from build123d import *

# Parameters (mm, degrees)
F1_DEPTH = 5
F2_W     = 5
F2_H     = 40
F3_DEPTH = 12
F4_R     = 3
F5_R     = 1.5
F6_DEPTH = 10


with BuildPart() as f1:
    # F0 (on Top) → F1 (new body)
    with BuildSketch(Plane.XY):
        with BuildLine():
            ThreePointArc((-7.71248, 8.530396), (11.5, 0), (-7.71248, -8.530396))
            ThreePointArc((-7.71248, -8.530396), (-8.179899, -8.293039), (-8.703171, -8.324766))
            Line((-8.703171, -8.324766), (-13.541093, -9.959054))
            ThreePointArc((-13.541093, -9.959054), (-14.18276, -10.632379), (-13.992452, -11.54281))
            ThreePointArc((-13.992452, -11.54281), (2.75234, -17.929021), (16.810487, -6.814154))
            ThreePointArc((16.810487, -6.814154), (18.174589, -6.14164), (19.677769, -5.910335))
            Line((19.677769, -5.910335), (30.5, -5.910335))
            ThreePointArc((30.5, -5.910335), (34.035534, -7.374801), (35.5, -10.910335))
            Line((35.5, -10.910335), (35.5, -18))
            ThreePointArc((35.5, -18), (36.085786, -19.414214), (37.5, -20))
            Line((37.5, -20), (45.5, -20))
            Line((45.5, -20), (45.5, 0))
            Line((45.5, 0), (45.5, 20))
            Line((45.5, 20), (37.5, 20))
            ThreePointArc((37.5, 20), (36.085786, 19.414214), (35.5, 18))
            Line((35.5, 18), (35.5, 10.910335))
            ThreePointArc((35.5, 10.910335), (34.035534, 7.374801), (30.5, 5.910335))
            Line((30.5, 5.910335), (19.677769, 5.910335))
            ThreePointArc((19.677769, 5.910335), (18.174589, 6.14164), (16.810487, 6.814154))
            ThreePointArc((16.810487, 6.814154), (2.75234, 17.929021), (-13.992452, 11.54281))
            ThreePointArc((-13.992452, 11.54281), (-14.18276, 10.632379), (-13.541093, 9.959054))
            Line((-13.541093, 9.959054), (-8.703171, 8.324766))
            ThreePointArc((-8.703171, 8.324766), (-8.179899, 8.293039), (-7.71248, 8.530396))
        make_face()
    extrude(amount=F1_DEPTH)

    # F2 (on face) → F3 (join)
    with BuildSketch(Plane.XY.offset(5)):
        with Locations((43, 0)):
            Rectangle(F2_W, F2_H)
    extrude(amount=F3_DEPTH)

    # F4
    f4_edges = [f1.edges().sort_by_distance(p)[0] for p in [
        (40.5, 0, 5),
        (43, 20, 17),
        (43, -20, 17),
    ]]
    fillet(f4_edges, radius=F4_R)

    # F5 (on face) → F6 (cut)
    with BuildSketch(Plane(origin=(40.5, 0, 0), x_dir=(0, -1, 0), z_dir=(-1, 0, 0))):
        with Locations((-11.877556, 12)):
            Circle(F5_R)
        with Locations((11.877556, 12)):
            Circle(F5_R)
    extrude(amount=-F6_DEPTH, mode=Mode.SUBTRACT)


solid = f1.part
Geometry: final body of the model. Coordinates: model frame, mm. A direction names the side the tool comes from. Give positions to 0.01 mm unless a question says otherwise; leave off trailing zeros. Loops run counter-clockwise (first coordinate to the right, second up) from the corner with the lowest first, then second, coordinate; pieces in that order, holes last. Notation, with made-up numbers: (69, 3) -> (103, 3) arc R34 cw to (103, 33) -> close; hole circle Ø11 at (44, -17.75). An arc over 180 degrees is marked (long way). Put each result on its own line as item: value.
1. Pin query (flat end, axial travel): P1, Ø4, axis at x = 26, z = 2, coming from the -Y side; P2, Ø4, axis at y = 15.5, z = 3.5, coming from the -X side; P3, Ø10, axis at x = 26, y = 16, coming from the -Z side; P4, Ø4.5, axis at y = 9, z = 14, coming from the -X side. Return the tip coordinate at first contact, or that it passes through.
Taken from the geometry:
P1: stops at y = -5.91
P2: stops at x = -12.12
P3: passes through
P4: stops at x = 40.5
2. Cut plane C-C (y = 0). Return the cut outline in (x, z), plus the area to 3 significant figures.
Taken from the geometry:
outline: (11.5, 0) -> (45.5, 0) -> (45.5, 17) -> (40.5, 17) -> (40.5, 8) arc R3 cw to (37.5, 5) -> (11.5, 5) -> close
area: 232 mm2
3. Pull-direction query (X, two-part tool) for faces 5 (the cylindrical face through (34.07, 7.41, 2.46)), 6 (the cylindrical face through (39.64, 0.28, 5.9)), 7 (the cylindrical face through (42.965, 13.376, 12.066)); classes: released by +X, released by -X, zero draft, split by the parting line, or undercut.
Taken from the geometry:
face 5: undercut
face 6: released by -X
face 7: zero draft
4. Set-up query: faces 1 (the flat face through (42, -20, 7)), 2 (the flat face through (25, -5.91, 2)), 3 (the cylindrical face through (18.195, 6.135, 2.465)), 4 (the flat face through (-11.156, 9.153, 2.465)). Return all of +Z, -Z, +X, -X, +Y, -Y with unobstructed straight access to the full face (end or side cutting, diameter ignored); none if empty.
Taken from the geometry:
face 1: +Z, -Z, +X, -X, -Y
face 2: +Z, -Z, -Y
face 3: +Z, -Z, +Y
face 4: +Z, -Z, -X
5. Cut plane D-D (z = 2.25). Return the cut outline in (x, y).
Taken from the geometry:
outline: (-13.99, -11.54) arc R18.14 ccw to (16.81, -6.81) arc R5 cw to (19.68, -5.91) -> (30.5, -5.91) arc R5 cw to (35.5, -10.91) -> (35.5, -18) arc R2 ccw to (37.5, -20) -> (45.5, -20) -> (45.5, 20) -> (37.5, 20) arc R2 ccw to (35.5, 18) -> (35.5, 10.91) arc R5 cw to (30.5, 5.91) -> (19.68, 5.91) arc R5 cw to (16.81, 6.81) arc R18.14 ccw to (-13.99, 11.54) arc R1 ccw to (-13.54, 9.96) -> (-8.7, 8.32) arc R1 ccw to (-7.71, 8.53) arc R11.5 cw (long way) to (-7.71, -8.53) arc R1 ccw to (-8.7, -8.32) -> (-13.54, -9.96) arc R1 ccw to start
6. Ray query, line 1 along X through (y, z) = (10, 14); line 2 along X through (y, z) = (-0.5, 3); line 3 along Z through (x, y) = (8.5, 12). Return the intervals inside material, ascending. Write a range as [from, to].
Taken from the geometry:
line 1: x = [40.5, 45.5]
line 2: x = [11.49, 45.5]
line 3: z = [0, 5]
7. Cut plane B-B (x = 0). Return the cut outline in (y, z).
Taken from the geometry:
outline: (-18.14, 0) -> (-11.5, 0) -> (-11.5, 5) -> (-18.14, 5) -> close; (11.5, 0) -> (18.14, 0) -> (18.14, 5) -> (11.5, 5) -> close
8. Cut plane A-A (z = 12). Return the cut outline in (x, y), plus the area to 3 significant figures.
Taken from the geometry:
outline: (40.5, -20) -> (45.5, -20) -> (45.5, -13.38) -> (40.5, -13.38) -> close; (40.5, -10.38) -> (45.5, -10.38) -> (45.5, 10.38) -> (40.5, 10.38) -> close; (40.5, 13.38) -> (45.5, 13.38) -> (45.5, 20) -> (40.5, 20) -> close
area: 170 mm2
